Source: CAD feature listing. Evaluate the final solid. Frame: model axes, mm. Face numbers are marked on the shaded views. Give positions to 0.01 mm unless a question says otherwise; leave off trailing zeros. Order: outer loops, then holes, each group sorted by start corner. A loop starts at its lowest first (then second) coordinate and runs counter-clockwise, first axis right, second up. Notation, with made-up numbers: M -31.5,-12 L -22.5,-12 A35 ccw -22.5,21 Z; hole C 62,23 d9. An arc over 180 degrees is marked long. Answer in a Markdown table with one row per item. Add a question column.
(1) Section query A-A, the plane x = 0. Return loops of the section in (y, z).
(2) Section query D-D, the plane x = -3.75. Return loops of the section in (y, z).
(3) Pin query (flat end, axial travel): P1, Ø0.9, axis at x = 0, y = 0.5, coming from the +Z side; P2, Ø6, axis at x = -1, y = 2, coming from the -Z side; P3, Ø1.5, axis at y = -3, z = 3, coming from the +X side. Return the tip coordinate at first contact, or that it passes through.
(4) Mould query, pull axis X, two halves, no side actions, for the marked faces 1, 2 and 3. Classes: pulls with the +X half, pulls with the -X half, needs draft (parallel to the pull), parting line crosses it, or undercut.
(5) Section query B-B, the plane y = 0. Return loops of the section in (x, z).
(6) Section query C-C, the plane z = 1.25. Return loops of the section in (x, y).
(7) Material intervals for line 1 along Y through (x, z) = (0, 8.55); line 2 along Z through (x, y) = (-0.5, -4.5); line 3 along X through (y, z) = (0.75, 5.5), sorted ascending.
from build123d import *

# Parameters (mm, degrees)
SKETCH_R     = 6
PAD_DEPTH    = 9.5
SKETCH001_R  = 1.5
POCKET_DEPTH = 2
SKETCH002_R  = 0.25
PAD001_DEPTH = 3.5


with BuildPart() as part:
    # Sketch → Pad (new body)
    with BuildSketch(Plane.XY):
        Circle(SKETCH_R)
    extrude(amount=PAD_DEPTH)

    # Sketch001 (on Face3 of Pad) → Pocket (cut)
    with BuildSketch(Plane.XY.offset(9.5)):
        Circle(SKETCH001_R)
    extrude(amount=-POCKET_DEPTH, mode=Mode.SUBTRACT)

    # Sketch002 (on Face2 of Pocket) → Pad001 (join)
    with BuildSketch(Plane(origin=(0, 0, 0), x_dir=(1, 0, 0), z_dir=(0, 0, -1))):
        with Locations((-3.81, 0)):
            Circle(SKETCH002_R)
        with Locations((3.81, 0)):
            Circle(SKETCH002_R)
    extrude(amount=PAD001_DEPTH)


solid = part.part
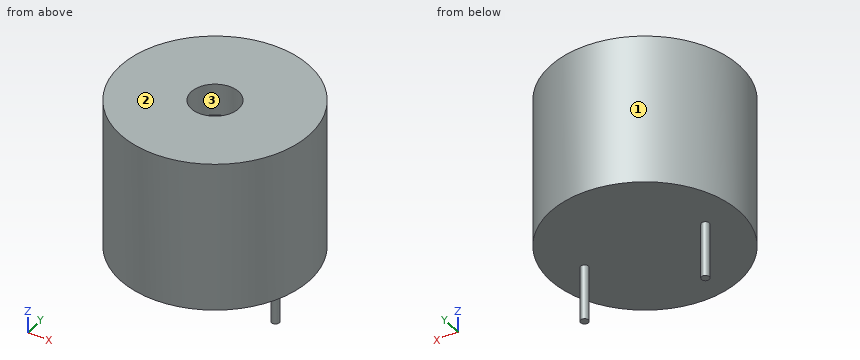
Values follow:
| question | item | result |
|---|---|---|
| 1 | outline | M -6,0 L 6,0 L 6,9.5 L 1.5,9.5 L 1.5,7.5 L -1.5,7.5 L -1.5,9.5 L -6,9.5 Z |
| 2 | outline | M -4.68,0 L -0.24,0 L -0.24,-3.5 L 0.24,-3.5 L 0.24,0 L 4.68,0 L 4.68,9.5 L -4.68,9.5 Z |
| 3 | P1 | stops at z = 7.5 |
| 3 | P2 | stops at z = 0 |
| 3 | P3 | stops at x = 5.56 |
| 4 | face 1 | parting line crosses it |
| 4 | face 2 | needs draft |
| 4 | face 3 | undercut |
| 5 | outline | M -6,0 L -4.06,0 L -4.06,-3.5 L -3.56,-3.5 L -3.56,0 L 3.56,0 L 3.56,-3.5 L 4.06,-3.5 L 4.06,0 L 6,0 L 6,9.5 L 1.5,9.5 L 1.5,7.5 L -1.5,7.5 L -1.5,9.5 L -6,9.5 Z |
| 6 | outline | C 0,0 d12 |
| 7 | line 1 | y = -6 to -1.5, 1.5 to 6 |
| 7 | line 2 | z = 0 to 9.5 |
| 7 | line 3 | x = -5.95 to 5.95 |
